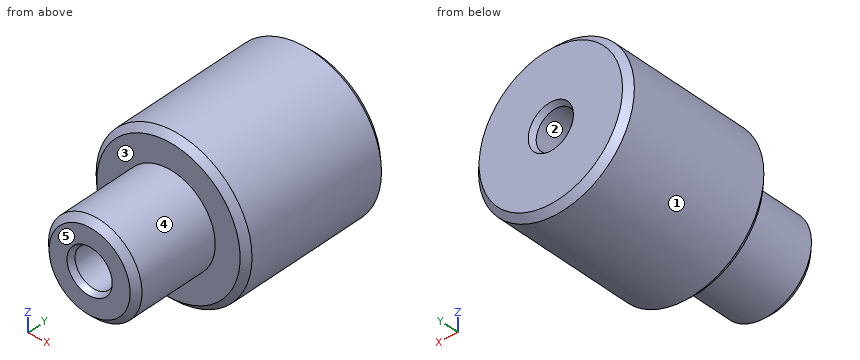
from build123d import *
from OCP.BRepFilletAPI import BRepFilletAPI_MakeChamfer

# Parameters (mm, degrees)
CHAMFER1_SIZE                = 2
F_12_5_12_5_DIAMETER_HOLE1_D = 12.5
CHAMFER2_SIZE                = 1
CHAMFER2_SIZE2               = 1.732050808


with BuildPart() as part:
    # Sketch1 → Revolve1 (revolve)
    with BuildSketch(Plane.XY, mode=Mode.PRIVATE) as revolve1_sk:
        Polygon((0, 0), (25, 0), (25, -50), (15, -50), (15, -78), (0, -78), align=None)
    revolve(revolve1_sk.sketch.rotate(Axis((0, 5, 0), (0, -1, 0)), 180), axis=Axis((0, 5, 0), (0, -1, 0)))

    # Chamfer1
    chamfer1_edges = [part.edges().sort_by_distance(p)[0] for p in [
        (15, -78, 0),
        (25, -50, 0),
        (25, 0, 0),
    ]]
    chamfer(chamfer1_edges, length=CHAMFER1_SIZE)

    # Ø12.5 (12.5) Diameter Hole1 (through all)
    with Locations(Plane(origin=(0, 0, 0), x_dir=(1, 0, 0), z_dir=(0, 1, 0))):
        with Locations((0, 0)):
            Hole(F_12_5_12_5_DIAMETER_HOLE1_D / 2)

    # Chamfer2: one chamfer whose edges measure the first distance from different faces: ONE call of the kernel's chamfer builder (chamfer() names one face for all edges)
    chamfer2_edges_1 = [part.edges().sort_by_distance(p)[0] for p in [
        (6.25, 0, 0),
    ]]
    chamfer2_side_1 = [part.faces().sort_by_distance(p)[0] for p in [
        (22.349461761, 0, 0),
    ]]
    chamfer2_edges_2 = [part.edges().sort_by_distance(p)[0] for p in [
        (6.25, -78, 0),
    ]]
    chamfer2_side_2 = [part.faces().sort_by_distance(p)[0] for p in [
        (12.632304474, -78, 0),
    ]]
    chamfer2 = BRepFilletAPI_MakeChamfer(part.part.solid().wrapped)
    for e in chamfer2_edges_1:
        chamfer2.Add(CHAMFER2_SIZE, CHAMFER2_SIZE2, e.wrapped, chamfer2_side_1[0].wrapped)  # the first distance lies on this face
    for e in chamfer2_edges_2:
        chamfer2.Add(CHAMFER2_SIZE, CHAMFER2_SIZE2, e.wrapped, chamfer2_side_2[0].wrapped)  # the first distance lies on this face
    add(Compound.cast(chamfer2.Shape()), mode=Mode.REPLACE)


solid = part.part
Input: part model. Units: mm. Frame: model coordinates. Face numbers are marked on the shaded views. A direction names the side the tool comes from. Give positions to 0.01 mm unless a question says otherwise; leave off trailing zeros. Loops run counter-clockwise (first coordinate to the right, second up) from the corner with the lowest first, then second, coordinate; pieces in that order, holes last. Notation, with made-up numbers: (-21.5, 12) - (6.5, 12) arc R28 cw to (6.5, 39) - close; hole circle Ø8 at (86.5, 50.25). An arc over 180 degrees is marked (long way). Use CSV: the item, a comma, the result in double quotes. Start each with the question number.
Item 1: Section C-C on y = -12.5. Return loops of the section in (x, z).
Item 2: Contact query for flat-ended pins moving along their axis: P1, Ø3, axis at x = -2, y = -67, coming from the +Z side; P2, Ø4, axis at y = -13.5, z = -10, coming from the -X side; P3, Ø2, axis at y = -21, z = -8, coming from the -X side. Output: stop coordinate, or through.
Item 3: Mould query, pull axis Z, two halves, no side actions, for the marked faces 1, 2 and 3. Classes: pulls with the +Z half, pulls with the -Z half, needs draft (parallel to the pull), parting line crosses it, or undercut.
Item 4: Line query: line 1 (Y direction, x = 18.5, z = 12); line 2 (Z direction, x = 0, y = -20.5); line 3 (Z direction, x = -5, y = -14). Output: solid intervals per line, ascending.
Item 5: Section B-B on z = 0. Return loops of the section in (x, y).
Item 6: Reachability of the marked faces 4 and 5 from +Z, -Z, +X, -X, +Y, -Y: full face, straight path, thin tool, end or side. Return the list, or none.
Item 7: Section A-A on x = 0. Return loops of the section in (y, z).
Ans:
1,outline,"circle Ø50 at (0, 0); hole circle Ø12.5 at (0, 0)"
2,P1,"stops at z = 14.99"
2,P2,"stops at x = -23.69"
2,P3,"stops at x = -24"
3,face 1,"parting line crosses it"
3,face 2,"undercut"
3,face 3,"needs draft"
4,line 1,"y = -50 to 0"
4,line 2,"z = -25 to -6.25, 6.25 to 25"
4,line 3,"z = -24.49 to -3.75, 3.75 to 24.49"
5,outline,"(-25, -48) - (-23, -50) - (-15, -50) - (-15, -76) - (-13, -78) - (-7.25, -78) - (-6.25, -76.27) - (-6.25, -1.73) - (-7.25, 0) - (-23, 0) - (-25, -2) - close; (6.25, -76.27) - (7.25, -78) - (13, -78) - (15, -76) - (15, -50) - (23, -50) - (25, -48) - (25, -2) - (23, 0) - (7.25, 0) - (6.25, -1.73) - close"
6,face 4,"-Y"
6,face 5,"+Z, -Z, +X, -X, -Y"
7,outline,"(-78, -13) - (-76, -15) - (-50, -15) - (-50, -23) - (-48, -25) - (-2, -25) - (0, -23) - (0, -7.25) - (-1.73, -6.25) - (-76.27, -6.25) - (-78, -7.25) - close; (-78, 7.25) - (-76.27, 6.25) - (-1.73, 6.25) - (0, 7.25) - (0, 23) - (-2, 25) - (-48, 25) - (-50, 23) - (-50, 15) - (-76, 15) - (-78, 13) - close"
